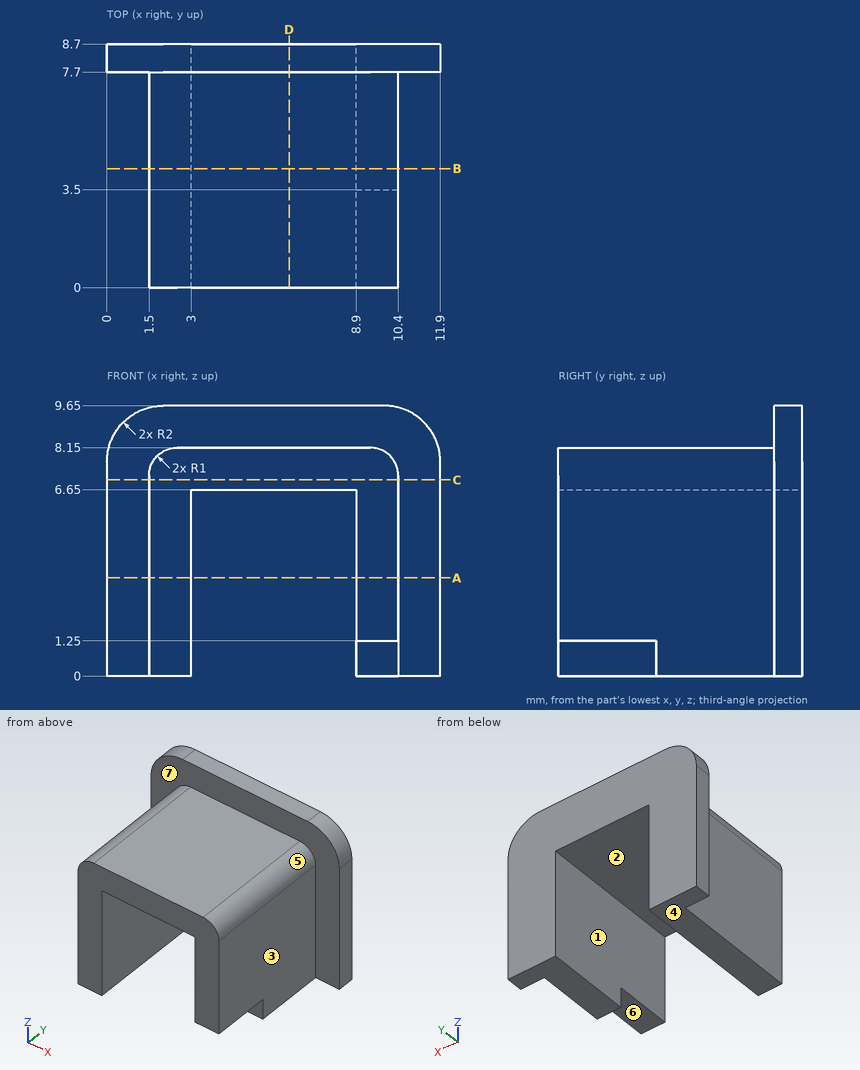
Design review of the part shown in the three views and the two pictorial views. Dimensions are in mm from the part's minimum x, y and z. A direction names the side the tool comes from. Coordinates: 2 decimals unless noted, no trailing zeros. Loops run counter-clockwise (first coordinate to the right, second up) from the corner with the lowest first, then second, coordinate; pieces in that order, holes last. Notation, with made-up numbers: M -2.5,39.25 L 54.5,39.25 A33 cw 54.5,74.25 Z; hole C 30,21 d3. An arc over 180 degrees is marked long. One line per question, with ' | ' between items.
(1) We need section C-C (z = 7). Give the boundary of the cut face in (x, y).
Filled in:
outline: M 0,7.7 L 1.5,7.7 L 1.5,0 L 10.4,0 L 10.4,7.7 L 11.9,7.7 L 11.9,8.7 L 0,8.7 Z
(2) Machinability: for the marked faces 5, 6 and 7, which of the approach directions +Z, -Z, +X, -X, +Y, -Y give a long, thin tool a straight path to every point of the face, cutting with its end or side? Answer none if there is none.
Filled in:
face 5: +Z, +X, -Y | face 6: -Z, +X, -Y | face 7: +Z, -Y
(3) We need section D-D (x = 6.5). Give the boundary of the cut face in (y, z).
Filled in:
outline: M 0,6.65 L 8.7,6.65 L 8.7,9.65 L 7.7,9.65 L 7.7,8.15 L 0,8.15 Z
(4) Draft analysis for pull direction X (two halves, no side actions). For the marked faces 1, 2, 3 and 4, state which applies: released by +X, released by -X, zero draft, split by the parting line, or undercut.
Filled in:
face 1: undercut | face 2: undercut | face 3: released by +X | face 4: zero draft
(5) We need section A-A (z = 3.5). Give the boundary of the cut face in (x, y).
Filled in:
outline: M 0,7.7 L 1.5,7.7 L 1.5,0 L 3,0 L 3,8.7 L 0,8.7 Z; M 8.9,0 L 10.4,0 L 10.4,7.7 L 11.9,7.7 L 11.9,8.7 L 8.9,8.7 Z
(6) For pin 1 Ø0.8 at (x, y) = (9.5, 1.5) entering from -Z; pin 2 Ø2 at (y, z) = (2, 7.5) entering from +X; pin 3 Ø2 at (y, z) = (2, 1.5) entering from -X, all flat-tipped, find the tip position at first contact; note any pin that passes through.
Filled in:
pin 1: stops at z = 1.25 | pin 2: stops at x = 10.4 | pin 3: stops at x = 1.5
(7) Wall thickness on probe 1 along X at (y, z) = (5, 1.25); probe 2 along X at (y, z) = (8, 3); probe 3 along X at (y, z) = (0.5, 6.75): over which ranges is each line inside the solid? List them lowest first.
Filled in:
probe 1: x = 1.5 to 3, 8.9 to 10.4 | probe 2: x = 0 to 3, 8.9 to 11.9 | probe 3: x = 1.5 to 10.4
(8) We need section B-B (y = 4.25). Give the boundary of the cut face in (x, z).
Filled in:
outline: M 1.5,0 L 3,0 L 3,6.65 L 8.9,6.65 L 8.9,0 L 10.4,0 L 10.4,7.15 A1 ccw 9.4,8.15 L 2.5,8.15 A1 ccw 1.5,7.15 Z
